Source: CAD feature listing. Evaluate the final solid. Frame: model axes, mm. A direction names the side the tool comes from. Give positions to 0.01 mm unless a question says otherwise; leave off trailing zeros. Order: outer loops, then holes, each group sorted by start corner. A loop starts at its lowest first (then second) coordinate and runs counter-clockwise, first axis right, second up. Notation, with made-up numbers: M 43,68.25 L 77,68.25 A25 ccw 77,93.25 Z; hole C 39,72 d5. An arc over 180 degrees is marked long. One line per question, with ' | ' between items. Start each with the question number.
from build123d import *

# Parameters (mm, degrees)
F1_DEPTH = 4
F2_W     = 7.5
F2_H     = 6
F3_DEPTH = 28
F4_R     = 2.99999
F2_R     = 1.5
F5_DEPTH = 25


# Not quite as in the source:
# - a fillet or chamfer is up to 0.001 mm smaller than in the source, because OpenCascade refuses the exact size


with BuildPart() as f1:
    # F0 (on Right) → F1 (new body)
    with BuildSketch(Plane.YZ):
        Polygon((-50, 55), (0, 55), (0, 65), (-18, 110), (-50, 110), align=None)
        Polygon((-50, 0), (-18, 0), (0, 45), (0, 55), (-50, 55), align=None)
        Polygon((-100, 55), (-50, 55), (-50, 110), (-82, 110), (-100, 65), align=None)
        Polygon((-82, 0), (-50, 0), (-50, 55), (-100, 55), (-100, 45), align=None)
    extrude(amount=F1_DEPTH)

    # F2 (on face) → F3 (join)
    with BuildSketch(Plane(origin=(0, 0, 0), x_dir=(0, -1, 0), z_dir=(-1, 0, 0))):
        with Locations((53.75, 7)):
            Rectangle(F2_W, F2_H)
        Polygon((42.5, 4), (50, 4), (50, 10), (42.5, 10), (42.5, 7), align=None)
    extrude(amount=F3_DEPTH)

    # F4 (radius 3 in the source; OpenCascade refuses exactly that, so slightly less here)
    f4_edges = [f1.edges().sort_by_distance(p)[0] for p in [
        (-28, -50, 4),
        (-28, -50, 10),
    ]]
    fillet(f4_edges, radius=F4_R)

    # F2 (on face) → F5 (cut)
    with BuildSketch(Plane(origin=(0, 0, 0), x_dir=(0, -1, 0), z_dir=(-1, 0, 0))):
        with Locations((72, 105)):
            Circle(F2_R)
        with Locations((85, 63)):
            Circle(F2_R)
        with Locations((85, 47)):
            Circle(F2_R)
        with Locations((15, 63)):
            Circle(F2_R)
        with BuildLine():
            ThreePointArc((16.5, 47), (15, 48.5), (13.5, 47))
            ThreePointArc((13.5, 47), (15, 45.5), (16.5, 47))
        make_face()
        with BuildLine():
            ThreePointArc((29.5, 105), (29.0606601718, 106.0606601718), (28, 106.5))
            ThreePointArc((28, 106.5), (26.9393398282, 103.9393398282), (29.5, 105))
        make_face()
        with Locations((63.5, 7)):
            Circle(F2_R)
        with Locations((36.5, 7)):
            Circle(F2_R)
    extrude(amount=-F5_DEPTH, mode=Mode.SUBTRACT)


solid = f1.part
Item 1: Reachability of faces 4 (the flat face through (-12, -50, 10)), 5 (the flat face through (2, 0, 55)), 6 (the flat face through (-12, -50, 4)) from +Z, -Z, +X, -X, +Y, -Y: full face, straight path, thin tool, end or side. Return the list, or none.
Item 2: Pin query (flat end, axial travel): pin 1 Ø10 at (x, y) = (-16, -45) entering from +Z; pin 2 Ø2.5 at (y, z) = (-63.5, 7) entering from +X; pin 3 Ø7.5 at (x, y) = (-10.5, -51) entering from -Z; pin 4 Ø6.5 at (x, z) = (-19, 6) entering from -Y. Return the tip coordinate at first contact, or that it passes through.
Item 3: Cut plane A-A on y = -85. Return the cut outline in (x, z).
Item 4: Cut plane D-D on x = -3. Return the cut outline in (y, z), and give its area (3 significant figures).
Item 5: Line query: line 1 (Z direction, x = 3.05, y = -36.5); line 2 (Z direction, x = 2.6, y = -72); line 3 (X direction, y = -80.5, z = 12.5). Output: solid intervals per line, ascending.
Item 6: Mould query, pull axis Z, two halves, no side actions, for faces 1 (the flat face through (2, -50, 0)), 2 (the cylindrical face through (1.972, -85.806, 64.265)), 3 (the cylindrical face through (-27.1, -49.9, 9.14)). Classes: pulls with the +Z half, pulls with the -Z half, needs draft (parallel to the pull), parting line crosses it, or undercut.
Item 7: Cut plane B-B on y = -72. Return the cut outline in (x, z).
Item 8: Cut plane C-C on z = 63. Return the cut outline in (x, y), and give its area (3 significant figures).
Results are:
1) face 4: +Z, -X, +Y, -Y | face 5: +Z, -Z, +X, -X, +Y | face 6: -Z, -X, +Y, -Y
2) pin 1: stops at z = 10 | pin 2: passes through | pin 3: stops at z = 4 | pin 4: stops at y = -57.5
3) outline: M 0,7.5 L 4,7.5 L 4,45.5 L 0,45.5 Z; M 0,48.5 L 4,48.5 L 4,61.5 L 0,61.5 Z; M 0,64.5 L 4,64.5 L 4,102.5 L 0,102.5 Z
4) outline: M -57.5,4 L -42.5,4 L -42.5,10 L -57.5,10 Z | area: 90.0 mm2
5) line 1: z = 0 to 5.5, 8.5 to 110 | line 2: z = 0 to 103.5, 106.5 to 110 | line 3: x = 0 to 4
6) face 1: pulls with the -Z half | face 2: undercut | face 3: pulls with the +Z half
7) outline: M 0,0 L 4,0 L 4,103.5 L 0,103.5 Z; M 0,106.5 L 4,106.5 L 4,110 L 0,110 Z
8) outline: M 0,-100 L 4,-100 L 4,-86.5 L 0,-86.5 Z; M 0,-83.5 L 4,-83.5 L 4,-16.5 L 0,-16.5 Z; M 0,-13.5 L 4,-13.5 L 4,0 L 0,0 Z | area: 376 mm2
